Here's the drawing with two shaded views (mm, measured from the low corner). I have some questions. A direction names the side the tool comes from. Coordinates: 2 decimals unless noted, no trailing zeros. Write each loop counter-clockwise with the first axis right and the second up, starting at its lowest first coordinate (ties: lowest second). Pieces come first, ordered by that corner, then holes. Notation, with made-up numbers: (47, 43.25) -> (81, 43.25) arc R18 cw to (81, 55.25) -> close; hole circle Ø10 at (70, 43.5). An arc over 180 degrees is marked (long way). Put each result on its own line as item: value. Start each with the question number.
Item 1: I want a section at A-A, the plane x = 19.75. State how many separate pieces and enclosed holes the cut face has, then the cut area to 4 significant figures.
Item 2: For pin 1 (3 mm diameter, centred on y = 14, z = 9.5, fed in from -X); pin 2 (6.5 mm diameter, centred on x = 19.75, y = 5.75, fed in from -Z); pin 3 (1.5 mm diameter, centred on y = 12, z = 15, fed in from -X), each with a flat end and sliding along its axis, tell me the tip position at first contact or that it passes through.
Item 3: If we mould it in two halves opening along X, with no side actions, what happens to the marked faces 4, 5 and 6? For each: released by +X, released by -X, zero draft, split by the parting line, or undercut.
Item 4: I want a section at B-B, the plane z = 8.25. List the corners of the cut face in (x, y) for me, then the cut area to 3 significant figures.
Item 5: I need wall thicknesses on line 1 (Y direction, x = 19.75, z = 15.9); line 2 (X direction, y = 19.5, z = 3.25); line 3 (Y direction, x = 19.75, z = 5.5). Which ranges of each line are inside material? Lowest first, please. Write a range as [from, to].
Item 6: On a 3-axis mill with a long thin cutter (end or side, diameter ignored), from which of +Z, -Z, +X, -X, +Y, -Y can I reach the whole of each face in a straight line? I mean the marked faces 1, 2 and 3. Say none if no direction works.
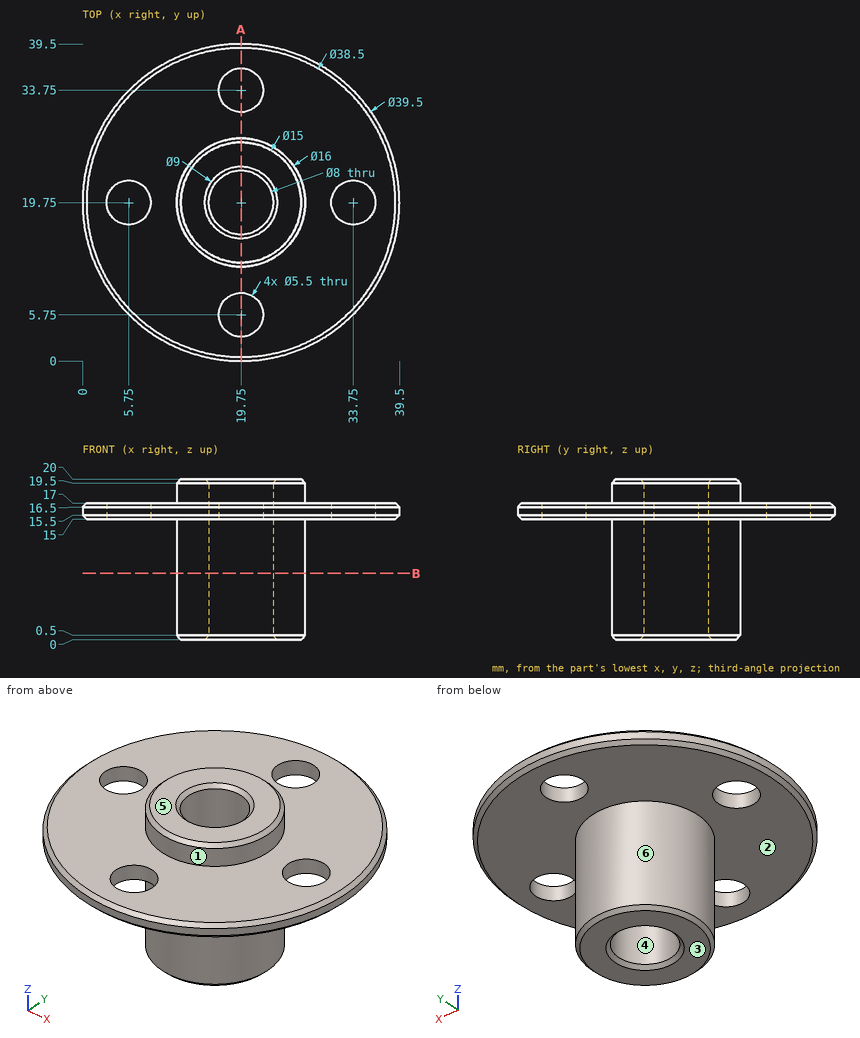
Calculated:
1. separate pieces: 4
1. enclosed holes: 0
1. area: 183.5 mm2
2. pin 1: stops at x = 12.97
2. pin 2: stops at z = 15
2. pin 3: stops at x = 1.36
3. face 4: undercut
3. face 5: zero draft
3. face 6: split by the parting line
4. outline: circle Ø16 at (19.75, 19.75); hole circle Ø8 at (19.75, 19.75)
4. area: 151 mm2
5. line 1: y = [0, 3], [8.5, 15.75], [23.75, 31], [36.5, 39.5]
5. line 2: x = [11.75, 15.76], [23.74, 27.75]
5. line 3: y = [11.75, 15.75], [23.75, 27.75]
6. face 1: +Z
6. face 2: -Z
6. face 3: -Z, +X, -X, +Y, -Y
